Here's how the part is built. I have some questions about the finished solid (model axes, mm). Face numbers are marked on the shaded views. A direction names the side the tool comes from. Round coordinates to 2 decimals unless told otherwise and drop trailing zeros. Order: outer loops, then holes, each group sorted by start corner. A loop starts at its lowest first (then second) coordinate and runs counter-clockwise, first axis right, second up.
```python
from build123d import *

# Parameters (mm, degrees)
BOSS_EXTRUDE1_DEPTH = 100
SKETCH2_W           = 40
SKETCH2_H           = 70
CUT_EXTRUDE1_DEPTH  = 100
SKETCH3_R           = 2.35
CUT_EXTRUDE2_DEPTH  = 6
CUT_EXTRUDE3_REACH  = 127.714
SKETCH4_R           = 1.5
SKETCH4_W           = 41
SKETCH4_H           = 21
SKETCH5_R           = 2.35
CUT_EXTRUDE4_DEPTH  = 6
SKETCH6_R           = 2.35
CUT_EXTRUDE5_DEPTH  = 6
CUT_EXTRUDE6_START  = -6
SKETCH7_R           = 2.35
CUT_EXTRUDE6_DEPTH  = 6
FILLET2_R           = 2


with BuildPart() as part:
    # Sketch1 → Boss-Extrude1 (new body)
    with BuildSketch(Plane.XY):
        Polygon((0, 46.3), (0, 0), (70, 0), (70, 8), (9.5, 8), (9.5, 38.3), (70, 38.3), (70, 46.3), align=None)
    extrude(amount=BOSS_EXTRUDE1_DEPTH)

    # Sketch2 → Cut-Extrude1 (cut)
    with BuildSketch(Plane.XZ):
        with Locations((35, 50)):
            Rectangle(SKETCH2_W, SKETCH2_H)
    extrude(amount=-CUT_EXTRUDE1_DEPTH, mode=Mode.SUBTRACT)

    # Sketch3 → Cut-Extrude2 (cut)
    with BuildSketch(Plane(origin=(70, 0, 0), x_dir=(0, 0, -1), z_dir=(1, 0, 0))):
        with Locations((-96, 42.3)):
            Circle(SKETCH3_R)
        with Locations(Location((-4, 42.3, 0), (0, 0, 180))):
            Circle(SKETCH3_R)
        with Locations((-4, 4)):
            Circle(SKETCH3_R)
        with Locations(Location((-96, 4, 0), (0, 0, 180))):
            Circle(SKETCH3_R)
    extrude(amount=-CUT_EXTRUDE2_DEPTH, mode=Mode.SUBTRACT)

    # Sketch4 → Cut-Extrude3 (cut, up to next)
    with BuildSketch(Plane(origin=(9.5, 0, 0), x_dir=(0, 0, -1), z_dir=(1, 0, 0)), mode=Mode.PRIVATE) as cut_extrude3_sk1:
        with Locations((-95.5, 28.15)):
            Circle(SKETCH4_R)
    cut_extrude3_tool1 = extrude(cut_extrude3_sk1.sketch, amount=-CUT_EXTRUDE3_REACH, mode=Mode.PRIVATE) & part.part
    # Sketch4 → Cut-Extrude3 (cut, up to next)
    with BuildSketch(Plane(origin=(9.5, 0, 0), x_dir=(0, 0, -1), z_dir=(1, 0, 0)), mode=Mode.PRIVATE) as cut_extrude3_sk2:
        with Locations((-95.5, 18.15)):
            Circle(SKETCH4_R)
    cut_extrude3_tool2 = extrude(cut_extrude3_sk2.sketch, amount=-CUT_EXTRUDE3_REACH, mode=Mode.PRIVATE) & part.part
    # Sketch4 → Cut-Extrude3 (cut, up to next)
    with BuildSketch(Plane(origin=(9.5, 0, 0), x_dir=(0, 0, -1), z_dir=(1, 0, 0)), mode=Mode.PRIVATE) as cut_extrude3_sk3:
        with Locations((-47.5, 18.15)):
            Circle(SKETCH4_R)
    cut_extrude3_tool3 = extrude(cut_extrude3_sk3.sketch, amount=-CUT_EXTRUDE3_REACH, mode=Mode.PRIVATE) & part.part
    # Sketch4 → Cut-Extrude3 (cut, up to next)
    with BuildSketch(Plane(origin=(9.5, 0, 0), x_dir=(0, 0, -1), z_dir=(1, 0, 0)), mode=Mode.PRIVATE) as cut_extrude3_sk4:
        with Locations((-47.5, 28.15)):
            Circle(SKETCH4_R)
    cut_extrude3_tool4 = extrude(cut_extrude3_sk4.sketch, amount=-CUT_EXTRUDE3_REACH, mode=Mode.PRIVATE) & part.part
    # Sketch4 → Cut-Extrude3 (cut, up to next)
    with BuildSketch(Plane(origin=(9.5, 0, 0), x_dir=(0, 0, -1), z_dir=(1, 0, 0)), mode=Mode.PRIVATE) as cut_extrude3_sk5:
        with Locations((-71.5, 23.15)):
            Rectangle(SKETCH4_W, SKETCH4_H)
    cut_extrude3_tool5 = extrude(cut_extrude3_sk5.sketch, amount=-CUT_EXTRUDE3_REACH, mode=Mode.PRIVATE) & part.part
    add(cut_extrude3_tool1.solids().sort_by_distance((9.5, 28.15, 95.5))[0], mode=Mode.SUBTRACT)
    add(cut_extrude3_tool2.solids().sort_by_distance((9.5, 18.15, 95.5))[0], mode=Mode.SUBTRACT)
    add(cut_extrude3_tool3.solids().sort_by_distance((9.5, 18.15, 47.5))[0], mode=Mode.SUBTRACT)
    add(cut_extrude3_tool4.solids().sort_by_distance((9.5, 28.15, 47.5))[0], mode=Mode.SUBTRACT)
    add(cut_extrude3_tool5.solids().sort_by_distance((9.5, 23.15, 71.5))[0], mode=Mode.SUBTRACT)

    # Sketch5 → Cut-Extrude4 (cut)
    with BuildSketch(Plane(origin=(0, 46.3, 0), x_dir=(1, 0, 0), z_dir=(0, 1, 0))):
        with Locations((4, -89)):
            Circle(SKETCH5_R)
        with Locations(Location((66, -89, 0), (0, 0, 180))):
            Circle(SKETCH5_R)
        with Locations((66, -11)):
            Circle(SKETCH5_R)
        with Locations(Location((4, -11, 0), (0, 0, 180))):
            Circle(SKETCH5_R)
    extrude(amount=-CUT_EXTRUDE4_DEPTH, mode=Mode.SUBTRACT)

    # Sketch6 → Cut-Extrude5 (cut)
    with BuildSketch(Plane.XY.offset(100)):
        with Locations((4, 4)):
            Circle(SKETCH6_R)
        with Locations((35, 4)):
            Circle(SKETCH6_R)
    extrude(amount=-CUT_EXTRUDE5_DEPTH, mode=Mode.SUBTRACT)

    # Sketch7 → Cut-Extrude6 (cut)
    with BuildSketch(Plane(origin=(0, 0, 0), x_dir=(-1, 0, 0), z_dir=(0, 0, -1)).offset(CUT_EXTRUDE6_START)):
        with Locations(Location((-35, 4, 0), (0, 0, 180))):
            Circle(SKETCH7_R)
        with Locations(Location((-4, 4, 0), (0, 0, 180))):
            Circle(SKETCH7_R)
    extrude(amount=CUT_EXTRUDE6_DEPTH, mode=Mode.SUBTRACT)

    # Fillet2
    # the kernel refuses this fillet: 2 mm, written as the material it takes off along each edge
    with BuildSketch(Plane(origin=(-5, 0, 0), x_dir=(0, 1, 0), z_dir=(1, 0, 0))) as fillet2_piece_1:
        with BuildLine():
            CenterArc((FILLET2_R, FILLET2_R), FILLET2_R, 180, 90)
            Line((0, FILLET2_R), (0, 0))
            Line((0, 0), (FILLET2_R, 0))
        make_face()
    extrude(amount=80, mode=Mode.SUBTRACT)
    with BuildSketch(Plane(origin=(0, 51.3, 0), x_dir=(0, 0, 1), z_dir=(0, -1, 0))) as fillet2_piece_2:
        with BuildLine():
            CenterArc((FILLET2_R, -FILLET2_R), FILLET2_R, 90, 90)
            Line((0, -FILLET2_R), (0, 0))
            Line((0, 0), (FILLET2_R, 0))
        make_face()
    extrude(amount=56.3, mode=Mode.SUBTRACT)
    with BuildSketch(Plane(origin=(75, 46.3, 0), x_dir=(0, 0, 1), z_dir=(-1, 0, 0))) as fillet2_piece_3:
        with BuildLine():
            CenterArc((FILLET2_R, -FILLET2_R), FILLET2_R, 90, 90)
            Line((0, -FILLET2_R), (0, 0))
            Line((0, 0), (FILLET2_R, 0))
        make_face()
    extrude(amount=80, mode=Mode.SUBTRACT)


solid = part.part
```
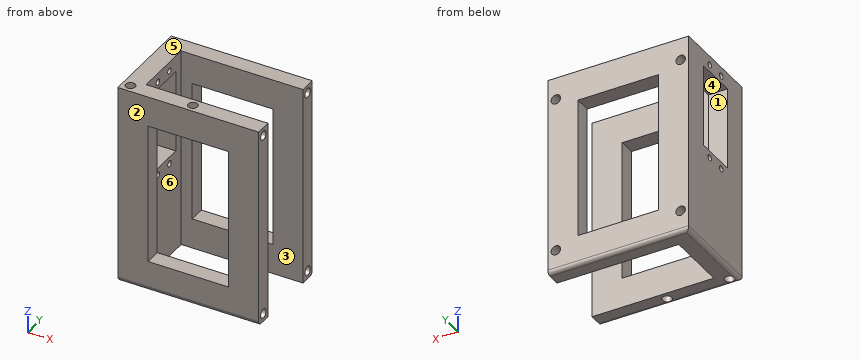
1. If we section it at B-B, the plane z = 89: Write out the boundary of the cut face in (x, y), and give its area (3 significant figures).
Evaluation:
outline: (0, 0) - (70, 0) - (70, 8) - (9.5, 8) - (9.5, 12.65) - (0, 12.65) - close; (0, 33.65) - (9.5, 33.65) - (9.5, 38.3) - (70, 38.3) - (70, 46.3) - (68.35, 46.3) - (68.35, 40.3) - (63.65, 40.3) - (63.65, 46.3) - (6.35, 46.3) - (6.35, 40.3) - (1.65, 40.3) - (1.65, 46.3) - (0, 46.3) - close
area: 1,150 mm2
2. If we section it at A-A, the plane y = 28.15: Write out the boundary of the cut face in (x, z), and give its area (3 significant figures).
Evaluation:
outline: (0, 2) arc R2 ccw to (2, 0) - (9.5, 0) - (9.5, 46) - (0, 46) - close; (0, 49) - (9.5, 49) - (9.5, 51) - (0, 51) - close; (0, 92) - (9.5, 92) - (9.5, 94) - (0, 94) - close; (0, 97) - (9.5, 97) - (9.5, 100) - (0, 100) - close
area: 503 mm2
3. I need wall thicknesses on probe 1 along Y at (x, z) = (35, 2.5); probe 2 along X at (y, z) = (4, 4); probe 3 along X at (y, z) = (42, 47). Which ranges of each line are inside material? Lowest first, please.
Evaluation:
probe 1: y = 0 to 1.65, 6.35 to 8, 38.3 to 46.3
probe 2: x = 0 to 1.65, 6.35 to 32.65, 37.35 to 64
probe 3: x = 0 to 15, 55 to 70
4. I'm going to push flat-ended pins straight in: P1, Ø2.5, axis at y = 42, z = 95, coming from the +X side; P2, Ø2.5, axis at x = 36, y = 4, coming from the +Z side; P3, Ø1.4, axis at x = 5, z = 89.5, coming from the +Y side. Where does each tip first touch, or does it pass through?
Evaluation:
P1: stops at x = 64
P2: stops at z = 94
P3: stops at y = 40.3
5. On a 3-axis mill with a long thin cutter (end or side, diameter ignored), from which of +Z, -Z, +X, -X, +Y, -Y can I reach the whole of each face in a straight line? I mean the marked faces 1, 2 and 3. Say none if no direction works.
Evaluation:
face 1: +X, -X
face 2: +Z, -Z, +X, -X, -Y
face 3: +Z, -Z, +X
6. If we mould it in two halves opening along Z, with no side actions, what happens to the marked faces 4, 5 and 6? For each: released by +Z, released by -Z, zero draft, split by the parting line, or undercut.
Evaluation:
face 4: undercut
face 5: released by +Z
face 6: zero draft
7. If we section it at C-C, the plane x = 30: Write out the boundary of the cut face in (y, z).
Evaluation:
outline: (0, 2) arc R2 ccw to (2, 0) - (8, 0) - (8, 15) - (0, 15) - close; (0, 85) - (8, 85) - (8, 100) - (0, 100) - close; (38.3, 0) - (44.3, 0) arc R2 ccw to (46.3, 2) - (46.3, 15) - (38.3, 15) - close; (38.3, 85) - (46.3, 85) - (46.3, 100) - (38.3, 100) - close
8. If we section it at D-D, the plane z = 47.5: Write out the boundary of the cut face in (x, y), and give its area (3 significant figures).
Evaluation:
outline: (0, 0) - (15, 0) - (15, 8) - (9.5, 8) - (9.5, 16.65) - (0, 16.65) - close; (0, 19.65) - (9.5, 19.65) - (9.5, 26.65) - (0, 26.65) - close; (0, 29.65) - (9.5, 29.65) - (9.5, 38.3) - (15, 38.3) - (15, 46.3) - (0, 46.3) - close; (55, 0) - (70, 0) - (70, 8) - (55, 8) - close; (55, 38.3) - (70, 38.3) - (70, 46.3) - (55, 46.3) - close
area: 711 mm2
